Input: part model. Units: mm. Frame: model coordinates. A direction names the side the tool comes from. Round coordinates to 2 decimals unless told otherwise and drop trailing zeros. Loops run counter-clockwise (first coordinate to the right, second up) from the corner with the lowest first, then second, coordinate; pieces in that order, holes last.
1) Draft query along Y for faces 3 (the face through (-3, 110, 10)), 4 (the face through (-3, -110, 10)), 5 (the face through (165, -1, 5)), 6 (the face through (180, -2, 10)). Return one class per face: pulls with the +Y half, pulls with the -Y half, needs draft (parallel to the pull), parting line crosses it, or undercut.
2) Section A-A, the plane z = 4. Return loops of the section in (x, y), and give its area (3 significant figures).
3) Access query for faces 1 (the face through (-180, -2, 10)), 2 (the face through (-170, 100, 5)). Directions: +Z, -Z, +X, -X, +Y, -Y. A direction counts if a zero-diameter tool reaches every point of the face in a straight line with its end or side. Return the directions, or none.
4) Section B-B, the plane y = -10.5. Return loops of the section in (x, z), and give its area (3 significant figures).
5) First-contact query: pin 1 (8 mm diameter, centred on x = 170.5, y = 44, fed in from -Z). Flat tip, straight axial feed; report the tip coordinate or a pass-through.
6) Ray query, line 1 along X through (y, z) = (5.5, 6.5). Return the intervals inside material, ascending.
from build123d import *

# Parameters (mm, degrees)
F0_W     = 360
F0_H     = 220
F1_DEPTH = 20
F2_W     = 10
F2_H     = 200
F3_DEPTH = 10
F4_W     = 10
F4_H     = 200
F5_DEPTH = 10


with BuildPart() as f1:
    # F0 (on Top) → F1 (new body)
    with BuildSketch(Plane.XY):
        Rectangle(F0_W, F0_H)
    extrude(amount=F1_DEPTH)

    # F2 (on Top) → F3 (cut)
    with BuildSketch(Plane.XY):
        with Locations((-170, 0)):
            Rectangle(F2_W, F2_H)
    extrude(amount=F3_DEPTH, mode=Mode.SUBTRACT)

    # F4 (on Top) → F5 (cut)
    with BuildSketch(Plane.XY):
        with Locations((170, 0)):
            Rectangle(F4_W, F4_H)
    extrude(amount=F5_DEPTH, mode=Mode.SUBTRACT)


solid = f1.part
Final values:
1. face 3: pulls with the +Y half
1. face 4: pulls with the -Y half
1. face 5: undercut
1. face 6: needs draft
2. outline: (-180, -110) - (180, -110) - (180, 110) - (-180, 110) - close; hole (-175, -100) - (-165, -100) - (-165, 100) - (-175, 100) - close; hole (165, -100) - (175, -100) - (175, 100) - (165, 100) - close
2. area: 75,200 mm2
3. face 1: +Z, -Z, -X, +Y, -Y
3. face 2: -Z
4. outline: (-180, 0) - (-175, 0) - (-175, 10) - (-165, 10) - (-165, 0) - (165, 0) - (165, 10) - (175, 10) - (175, 0) - (180, 0) - (180, 20) - (-180, 20) - close
4. area: 7,000 mm2
5. pin 1: stops at z = 10
6. line 1: x = -180 to -175, -165 to 165, 175 to 180
